```python
from build123d import *

# Parameters (mm, degrees)
SKETCH_2_R          = 2.5
CUT_EXTRUDE_1_DEPTH = 15.723805295


with BuildPart() as part:
    # Эскиз1 → Повернуть1 (revolve)
    with BuildSketch(Plane.XY):
        with BuildLine():
            Line((0, 0), (0, 6))
            Line((0, 6), (1, 6))
            Line((1, 6), (1, 3.5))
            Line((1, 3.5), (2, 3.5))
            Line((2, 3.5), (2, 4.5))
            ThreePointArc((2, 4.5), (7.361902647, 7), (12.723805295, 4.5))
            Line((12.723805295, 4.5), (12.723805295, 3.5))
            Line((12.723805295, 3.5), (13.723805295, 3.5))
            Line((13.723805295, 3.5), (13.723805295, 6))
            Line((13.723805295, 6), (14.723805295, 6))
            Line((14.723805295, 6), (14.723805295, 0))
            Line((14.723805295, 0), (11.723805295, 0))
            Line((11.723805295, 0), (11.723805295, 4.119927826))
            ThreePointArc((11.723805295, 4.119927826), (7.361902647, 6), (3, 4.119927826))
            Line((3, 4.119927826), (3, 0))
            Line((3, 0), (0, 0))
        make_face()
    revolve(axis=Axis((0, 0, 0), (1, 0, 0)))

    # Эскиз2 → Вырез-Вытянуть1 (cut, through all)
    with BuildSketch(Plane.ZY):
        Circle(SKETCH_2_R)
    extrude(amount=-CUT_EXTRUDE_1_DEPTH, mode=Mode.SUBTRACT)


solid = part.part
```
Geometry check sheet. Reference: the model listing, model coordinates, mm. A direction names the side the tool comes from. Coordinates: 2 decimals unless noted, no trailing zeros. Loops run counter-clockwise (first coordinate to the right, second up) from the corner with the lowest first, then second, coordinate; pieces in that order, holes last. Notation, with made-up numbers: (-13, 35.25) - (11, 35.25) arc R22 ccw to (11, 46.25) - close; hole circle Ø8 at (20.25, -3). An arc over 180 degrees is marked (long way). One line per item, written item: value. Start each with the question number.
(1) Mould release check, pull along Y, two halves, no side actions. Record for faces 1 (the flat face through (1, 3, -3)), 2 (the flat face through (11.724, -2, -2)), 3 (the cylindrical face through (14, -6, 0)): released by +Y, released by -Y, zero draft, split by the parting line, or undercut.
(2) Tool access check on faces 4 (the cylindrical face through (0.507, -5.994, 0.264)), 5 (the cylindrical face through (13.2, -2.44, -0.54)), 6 (the flat face through (2, 0, -4)). Record the directions out of +Z, -Z, +X, -X, +Y, -Y that give a thin tool (end or side, any length) a straight path to the whole face; none if there is none.
(3) Cross-section at D-D on x = 9.25. Enter the section's corners in (y, z).
(4) Cross-section at C-C on z = 2.75. Enter the section's corners in (x, y).
(5) Material ranges on line 1 (X direction, y = -1.25, z = -3.75); line 2 (X direction, y = -2.5, z = 5); line 3 (Z direction, x = 11, y = -0.5), recorded low to high. Write a range as [from, to].
(6) Depth check by flat-ended pin: P1, Ø6, axis at x = 12.5, y = 1, coming from the -Z side; P2, Ø3, axis at y = 0, z = 0, coming from the -X side; P3, Ø2, axis at x = 8, y = 2, coming from the -Z side; P4, Ø4, axis at x = 4, z = 5, coming from the -Y side. Enter the tip coordinate at first touch or a pass-through.
Results below:
1. face 1: zero draft
1. face 2: undercut
1. face 3: split by the parting line
2. face 4: -X
2. face 5: +X, -X
2. face 6: none
3. outline: circle Ø13.48 at (0, 0); hole circle Ø11.39 at (0, 0)
4. outline: (0, -5.33) - (1, -5.33) - (1, -2.17) - (2, -2.17) - (2, -3.56) arc R6.44 ccw to (12.72, -3.56) - (12.72, -2.17) - (13.72, -2.17) - (13.72, -5.33) - (14.72, -5.33) - (14.72, 5.33) - (13.72, 5.33) - (13.72, 2.17) - (12.72, 2.17) - (12.72, 3.56) arc R6.44 ccw to (2, 3.56) - (2, 2.17) - (1, 2.17) - (1, 5.33) - (0, 5.33) - close; hole (3, -3.07) arc R5.33 ccw to (11.72, -3.07) - (11.72, 3.07) arc R5.33 ccw to (3, 3.07) - close
5. line 1: x = [0, 1], [2, 3], [11.72, 12.72], [13.72, 14.72]
5. line 2: x = [0, 1], [3.15, 5.18], [9.54, 11.57], [13.72, 14.72]
5. line 3: z = [-5.96, -4.74], [4.74, 5.96]
6. P1: stops at z = -6.63
6. P2: passes through
6. P3: stops at z = -6.91
6. P4: stops at y = -5.73
